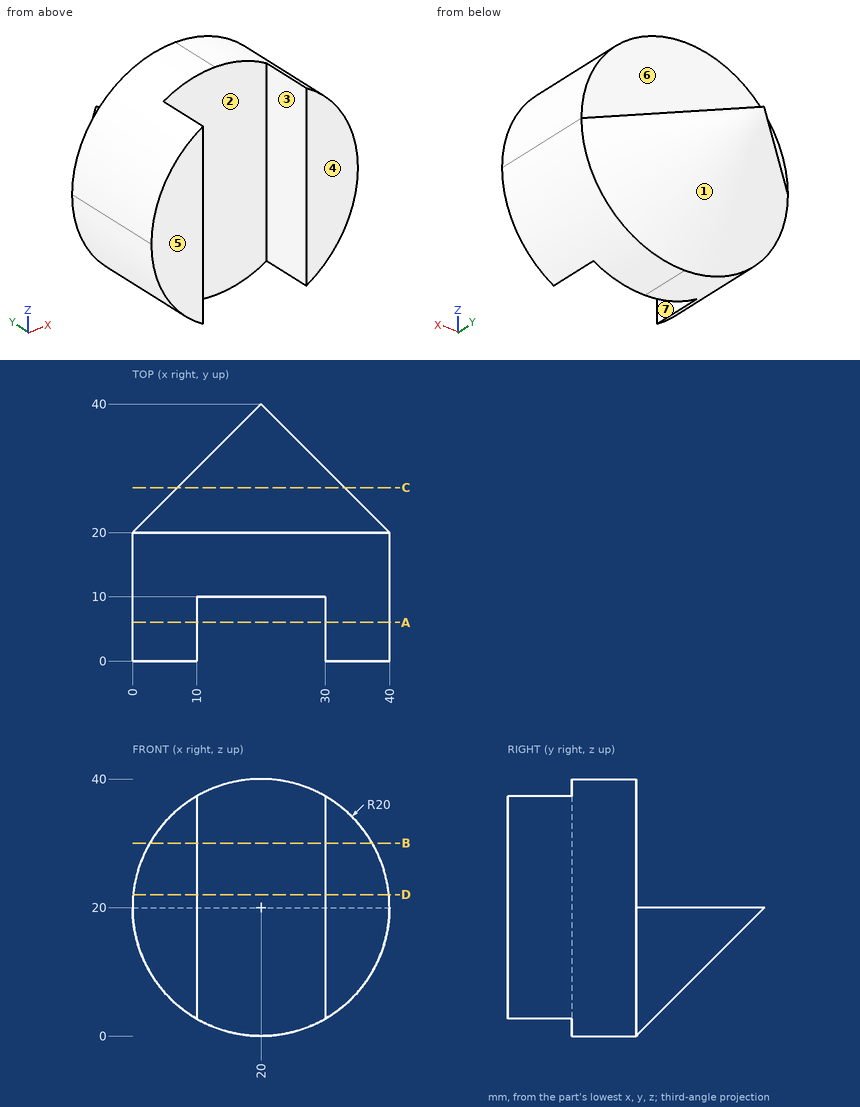
Geometry: see drawing. Coordinates: mm, zero at the bounding-box minimum. A direction names the side the tool comes from. Coordinates: 2 decimals unless noted, no trailing zeros. Loops run counter-clockwise (first coordinate to the right, second up) from the corner with the lowest first, then second, coordinate; pieces in that order, holes last.
(1) First-contact query: pin 1 Ø10 at (x, z) = (26, 34.5) entering from +Y; pin 2 Ø5 at (x, y) = (31, 24.5) entering from -Z; pin 3 Ø11 at (y, z) = (5.5, 11.5) entering from +X. Flat tips, straight axial feed; report the tip coordinate or a pass-through.
(2) Section C-C on y = 27. Return the cut outline in (x, z).
(3) Set-up query: the marked faces 5, 6 and 7. Return all of +Z, -Z, +X, -X, +Y, -Y with unobstructed straight access to the full face (end or side cutting, diameter ignored); none if empty.
(4) Section B-B on z = 30. Return the cut outline in (x, y), then the cut area to 3 significant figures.
(5) Section A-A on y = 6. Return the cut outline in (x, z), then the cut area to 3 significant figures.
(6) Material intervals for probe 1 along Y at (x, z) = (26.5, 30.5); probe 2 along Y at (x, z) = (30.5, 31.5); probe 3 along X at (y, z) = (17, 7), sorted ascending.
(7) Section D-D on z = 22. Return the cut outline in (x, y), then the cut area to 3 significant figures.
(8) Pull-direction query (X, two-part tool) for the marked faces 1, 2, 3 and 4; classes: released by +X, released by -X, zero draft, split by the parting line, or undercut.
Data:
1. pin 1: stops at y = 20
1. pin 2: stops at z = 5.27
1. pin 3: stops at x = 39.77
2. outline: (7, 20) arc R13 ccw to (33, 20) - close
3. face 5: +Z, -Z, +X, -X, -Y
3. face 6: +Z, +X, -X, +Y
3. face 7: +Z, -Z, -Y
4. outline: (2.68, 0) - (10, 0) - (10, 10) - (30, 10) - (30, 0) - (37.32, 0) - (37.32, 20) - (2.68, 20) - close
4. area: 493 mm2
5. outline: (10, 2.68) - (10, 37.32) arc R20 ccw to start; (30, 2.68) arc R20 ccw to (30, 37.32) - close
5. area: 491 mm2
6. probe 1: y = 10 to 20
6. probe 2: y = 0 to 20
6. probe 3: x = 4.8 to 35.2
7. outline: (0.1, 0) - (10, 0) - (10, 10) - (30, 10) - (30, 0) - (39.9, 0) - (39.9, 20) - (0.1, 20) - close
7. area: 596 mm2
8. face 1: split by the parting line
8. face 2: undercut
8. face 3: undercut
8. face 4: zero draft
